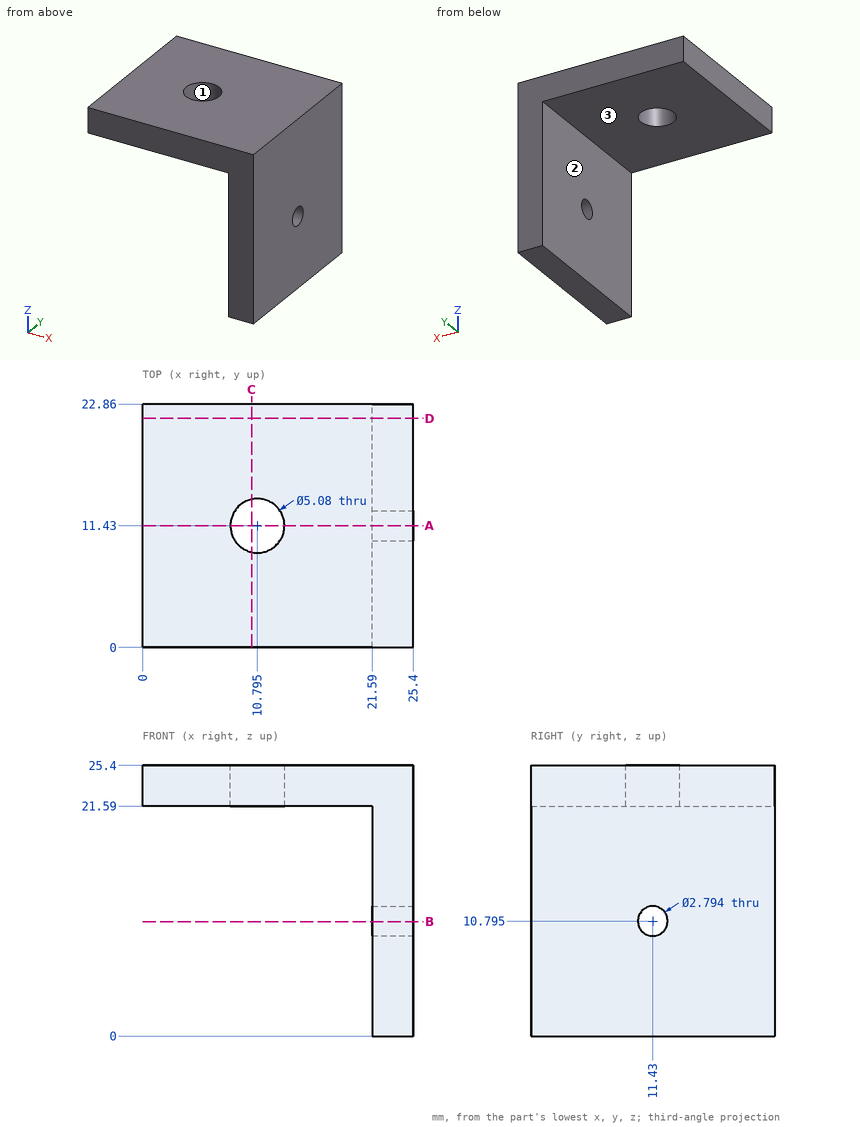
Source: three-view drawing plus pictorial views. Frame: mm from the lowest corner of the part. Round coordinates to 2 decimals unless told otherwise and drop trailing zeros. Write each loop counter-clockwise with the first axis right and the second up, starting at its lowest first coordinate (ties: lowest second). Pieces come first, ordered by that corner, then holes. Notation, with made-up numbers: M 46.25,14 L 87.25,14 A34 ccw 87.25,51 Z; hole C 63,-31 d2. An arc over 180 degrees is marked long. Use CSV: the item, a comma, the result in double quotes. Start each with the question number.
Q1. Cut plane B-B on z = 10.75. Output: boundary loops of the cut face in (x, y), plus the area to 3 significant figures.
Q2. Cut plane D-D on y = 21.5. Output: boundary loops of the cut face in (x, z), plus the area to 3 significant figures.
Q3. Pull-direction query (X, two-part tool) for the marked faces 1, 2 and 3; classes: +X half, -X half, draft (parallel to the pull), parting line (faces both ways), or undercut.
Q4. First-contact query: P1, Ø10, axis at x = 13.5, y = 17.5, coming from the -Z side; P2, Ø1.5, axis at x = 19.5, z = 12.5, coming from the +Y side; P3, Ø3, axis at y = 11.43, z = 10.795, coming from the -X side. Flat tips, straight axial feed; report the tip coordinate or a pass-through.
Q5. Line query: line 1 (Z direction, x = 23.2, y = 11.43); line 2 (X direction, y = 11.43, z = 23.6) (3 decimals); line 3 (X direction, y = 16, z = 7.75). Output: solid intervals per line, ascending. Write a range as from..to.
Q6. Cut plane C-C on x = 10.25. Output: boundary loops of the cut face in (y, z).
Q7. Cut plane A-A on y = 11.43. Output: boundary loops of the cut face in (x, z) (3 decimals), plus the area to 3 significant figures.
Results found:
1,outline,"M 21.59,0 L 25.4,0 L 25.4,10.03 L 21.59,10.03 Z; M 21.59,12.83 L 25.4,12.83 L 25.4,22.86 L 21.59,22.86 Z"
1,area,"76.5 mm^2"
2,outline,"M 0,21.59 L 21.59,21.59 L 21.59,0 L 25.4,0 L 25.4,25.4 L 0,25.4 Z"
2,area,"179 mm^2"
3,face 1,"undercut"
3,face 2,"-X half"
3,face 3,"draft"
4,P1,"z = 21.59"
4,P2,"through"
4,P3,"x = 21.59"
5,line 1,"0..9.4, 12.19..25.4"
5,line 2,"0..8.255, 13.335..25.4"
5,line 3,"21.59..25.4"
6,outline,"M 0,21.59 L 8.95,21.59 L 8.95,25.4 L 0,25.4 Z; M 13.91,21.59 L 22.86,21.59 L 22.86,25.4 L 13.91,25.4 Z"
7,outline,"M 0,21.59 L 8.255,21.59 L 8.255,25.4 L 0,25.4 Z; M 13.335,21.59 L 21.59,21.59 L 21.59,12.192 L 25.4,12.192 L 25.4,25.4 L 13.335,25.4 Z; M 21.59,0 L 25.4,0 L 25.4,9.398 L 21.59,9.398 Z"
7,area,"149 mm^2"
